Geometry check sheet. Reference: drawing and pictorial views, mm from the part's lowest x, y, z. Round coordinates to 2 decimals unless told otherwise and drop trailing zeros. Write each loop counter-clockwise with the first axis right and the second up, starting at its lowest first coordinate (ties: lowest second). Pieces come first, ordered by that corner, then holes. Notation, with made-up numbers: M 43.5,60 L 59.5,60 A12 ccw 59.5,69 Z; hole C -14.75,21 d4. An arc over 180 degrees is marked long. Answer in a Markdown table with one row per item. Add a question column.
1. Sectioned sample at A-A on y = 8.5. Record the cut outline in (x, z).
2. Sectioned sample at C-C on x = 10.5. Record the cut outline in (y, z).
3. Sectioned sample at B-B on z = 20.5. Record the cut outline in (x, y).
4. Sectioned sample at D-D on z = 3. Record the cut outline in (x, y).
5. Material ranges on probe 1 along Y at (x, z) = (21.5, 8.5); probe 2 along Z at (x, y) = (25, 21), recorded low to high.
6. Go/stop test with flat-tipped pins: pin 1 Ø12 at (x, z) = (42, 23) entering from +Y; pin 2 Ø6 at (y, z) = (6.5, 24) entering from +X; pin 3 Ø1.5 at (x, y) = (24.5, 18.5) entering from +Z. Record where each tip stops, or that it passes through.
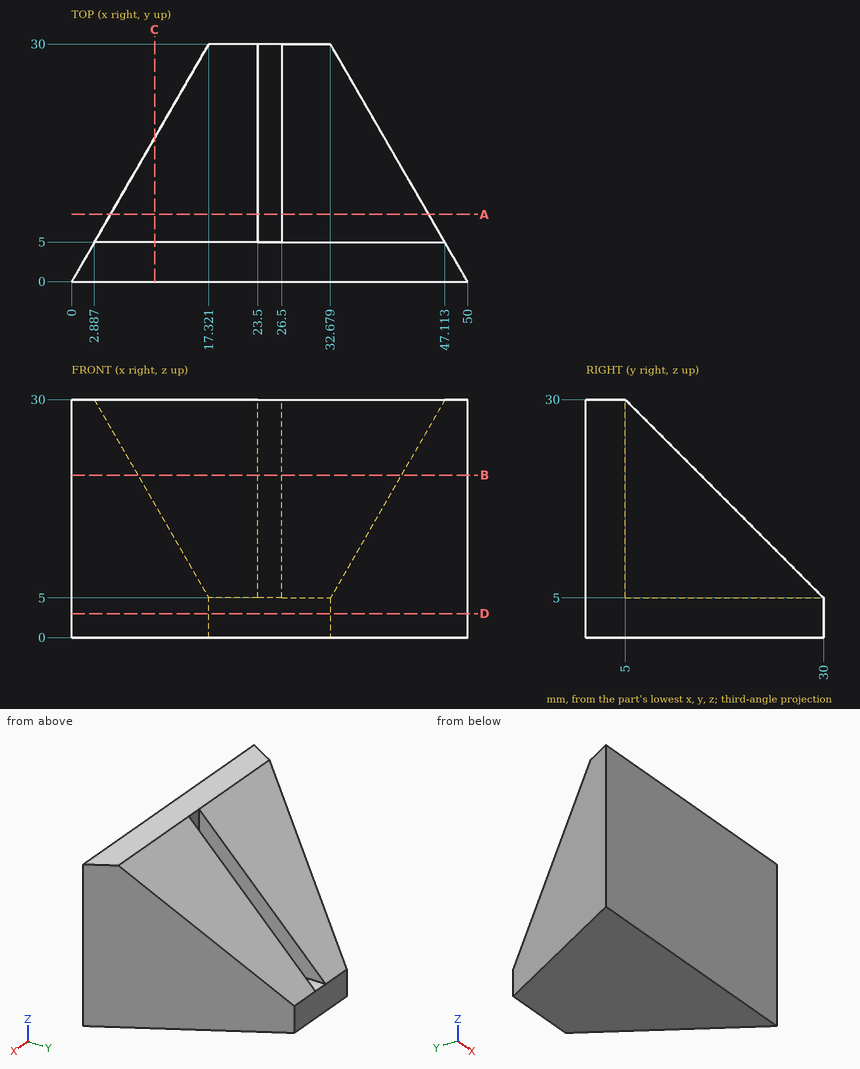
Geometry check:
| question | item | result |
|---|---|---|
| 1 | outline | M 4.91,0 L 45.09,0 L 45.09,26.5 L 26.5,26.5 L 26.5,5 L 23.5,5 L 23.5,26.5 L 4.91,26.5 Z |
| 2 | outline | M 0,0 L 18.19,0 L 18.19,16.81 L 5,30 L 0,30 Z |
| 3 | outline | M 0,0 L 50,0 L 41.63,14.5 L 26.5,14.5 L 26.5,5 L 23.5,5 L 23.5,14.5 L 8.37,14.5 Z |
| 4 | outline | M 0,0 L 50,0 L 32.68,30 L 17.32,30 Z |
| 5 | probe 1 | y = 0 to 26.5 |
| 5 | probe 2 | z = 0 to 5 |
| 6 | pin 1 | stops at y = 17.6 |
| 6 | pin 2 | stops at x = 47.98 |
| 6 | pin 3 | stops at z = 5 |
